Can you work these out from the model? Positions are in its coordinate system, mm. A direction names the side the tool comes from. Give positions to 0.01 mm unless a question says otherwise; leave off trailing zeros. Write each loop counter-clockwise with the first axis right and the second up, starting at its lowest first coordinate (ties: lowest second). Pieces come first, ordered by that corner, then holes.
1. On a 3-axis mill with a long thin cutter (end or side, diameter ignored), from which of +Z, -Z, +X, -X, +Y, -Y can I reach the whole of each face in a straight line? I mean faces 1 (the flat face through (11, 3, 0)), 2 (the flat face through (0, 3, -5.08)), 3 (the flat face through (-11, 3, 0)). Say none if no direction works.
2. Suppose I cut it at B-B (z = 9). Please give me the cut outline in (x, y), and give its area (3 significant figures).
3. Suppose I cut it at A-A (y = 1.95). Please give me the cut outline in (x, z), and give its area (3 significant figures).
4. If I drill on probe 1 along X at (y, z) = (1.8, -1.25); probe 2 along Z at (x, y) = (5, 0.9); probe 3 along X at (y, z) = (0.25, 6.75), over which ranges is the centre line in solid material (lowest first)?
5. I'm going to push flat-ended pins straight in: pin 1 (4 mm diameter, centred on x = 7, z = 6.5, fed in from -Y); pin 2 (1 mm diameter, centred on y = 1.5, z = 1.5, fed in from -X); pin 3 (2.5 mm diameter, centred on x = -9, y = 3.5, fed in from -Z); pin 4 (2 mm diameter, centred on x = -4.5, y = 3, fed in from +Z). Where does each tip first touch, or does it pass through?
6. Suppose I cut it at C-C (x = -12.25). Please give me the cut outline in (y, z).
```python
from build123d import *

# Parameters (mm, degrees)
SKETCH1_R           = 15
BOSS_EXTRUDE1_DEPTH = 5.08
SKETCH2_W           = 841.216063822
SKETCH2_H           = 769.249769976
CUT_EXTRUDE1_DEPTH  = 5.08
SKETCH3_W           = 12.7
SKETCH3_H           = 5.08
BOSS_EXTRUDE2_DEPTH = 5.08


with BuildPart() as part:
    # Sketch1 → Boss-Extrude1 (new body)
    with BuildSketch(Plane(origin=(0, 0, 0), x_dir=(1, 0, 0), z_dir=(0, 1, 0))):
        Circle(SKETCH1_R)
    extrude(amount=BOSS_EXTRUDE1_DEPTH)

    # Sketch2 → Cut-Extrude1 (cut)
    with BuildSketch(Plane(origin=(0, 5.08, 0), x_dir=(1, 0, 0), z_dir=(0, 1, 0))):
        with Locations((-405.608031911, 384.624884988)):
            Rectangle(SKETCH2_W, SKETCH2_H)
    extrude(amount=-CUT_EXTRUDE1_DEPTH, mode=Mode.SUBTRACT)

    # Sketch3 → Boss-Extrude2 (add)
    with BuildSketch(Plane(origin=(0, 0, 0), x_dir=(-1, 0, 0), z_dir=(0, 0, -1))):
        with Locations((0, 2.54)):
            Rectangle(SKETCH3_W, SKETCH3_H)
    extrude(amount=BOSS_EXTRUDE2_DEPTH)


solid = part.part
```
Checks:
1. face 1: -Z, +X, +Y, -Y
1. face 2: -Z, +X, -X, +Y, -Y
1. face 3: -Z, -X, +Y, -Y
2. outline: (-12, 0) - (12, 0) - (12, 5.08) - (-12, 5.08) - close
2. area: 122 mm2
3. outline: (-15, 0) - (-6.35, 0) - (-6.35, -5.08) - (6.35, -5.08) - (6.35, 0) - (15, 0) arc R15 ccw to start
3. area: 418 mm2
4. probe 1: x = -6.35 to 6.35
4. probe 2: z = -5.08 to 14.14
4. probe 3: x = -13.4 to 13.4
5. pin 1: stops at y = 0
5. pin 2: stops at x = -14.97
5. pin 3: stops at z = 0
5. pin 4: stops at z = 14.59
6. outline: (0, 0) - (5.08, 0) - (5.08, 8.66) - (0, 8.66) - close
